Geometry: final body of the model. Coordinates: model frame, mm. Face numbers are marked on the shaded views. A direction names the side the tool comes from. Give positions to 0.01 mm unless a question says otherwise; leave off trailing zeros. Order: outer loops, then holes, each group sorted by start corner. A loop starts at its lowest first (then second) coordinate and runs counter-clockwise, first axis right, second up. Notation, with made-up numbers: (71, -35.5) -> (80, -35.5) arc R16 ccw to (80, -25.5) -> close; hole circle Ø11 at (59, 69). An arc over 180 degrees is marked (long way). One line per question, with ' | ' between items.
Autodesk Inventor part; units mm, degrees
ref_plane "YZ Plane" through (0, 0, 0) normal (1, 0, 0) x (0, 1, 0)
ref_plane "XZ Plane" through (0, 0, 0) normal (0, 1, 0) x (-1, 0, 0)
ref_plane "XY Plane" through (0, 0, 0) normal (0, 0, 1) x (1, 0, 0)
sketch "Sketch1" plane through (0, 0, 0) normal (0, 1, 0) x (-1, 0, 0)
  line L0 (0, 0) -> (75, 0)
  line L1 (75, 0) -> (75, -75)
  line L2 (75, -75) -> (0, -75)
  line L3 (0, -75) -> (0, 0)
  dimension "d0" = 75
  dimension "d1" = 75
extrude "Extrusion1" add sketch "Sketch1" along normal blind 3.5
sketch "Sketch2" plane through (0, 3.5, 0) normal (0, 1, 0) x (1, 0, 0)
  line L0 (-75, 0) -> (0, 0)
  line L1 (0, 0) -> (0, 75)
  line L2 (0, 75) -> (-75, 75)
  line L3 (-75, 75) -> (-75, 0)
  line L4 (-75, 75) -> (-75, 0)
  line L5 (0, 0) -> (0, 75)
  line L6 (-5, 5) -> (-75, 5)
  line L7 (-70, 75) -> (-70, 0)
  circle A0 centre (-70, 37.5) radius 2.5
  circle A1 centre (-5, 37.5) radius 2.5
  line L8 (-75, 37.5) -> (-7.5, 37.5)
  line L9 (-2.5, 37.5) -> (0, 37.5)
  line L10 (-5, 75) -> (-5, 40)
  line L11 (-5, 35) -> (-5, 5)
  dimension "d5" = 5
  dimension "d6" = 5
  dimension "d7" = 5
extrude "Extrusion2" cut sketch "Sketch2" against normal blind 3.5 contours A0 L8 L7 | L7 L8 A0 | A0 L7 L8 | A1 | L7 A0 L8
sketch "Sketch3" plane through (0, 3.5, 0) normal (0, 1, 0) x (1, 0, 0)
  circle A0 centre (-70, 37.5) radius 2.5
  circle A1 centre (-5, 37.5) radius 2.5
  line L0 (-75, 0) -> (0, 0)
  line L1 (0, 0) -> (0, 75)
  line L2 (0, 75) -> (-75, 75)
  line L3 (-75, 75) -> (-75, 0)
  line L4 (-10, 10) -> (-10, 65)
  line L5 (-65, 65) -> (-65, 10)
  line L6 (-65, 65) -> (-65, 75)
  line L7 (0, 75) -> (-75, 75)
  line L8 (-65, 10) -> (-65, 0)
  line L9 (-75, 0) -> (0, 0)
  line L10 (-10, 10) -> (-10, 0)
  line L11 (-10, 65) -> (-10, 75)
  dimension "d10" = 10
extrude "Extrusion3" add sketch "Sketch3" along normal blind 32 contours L8 L5 L6 L2 L11 L4 L10 L0
properties part number "power_suply"
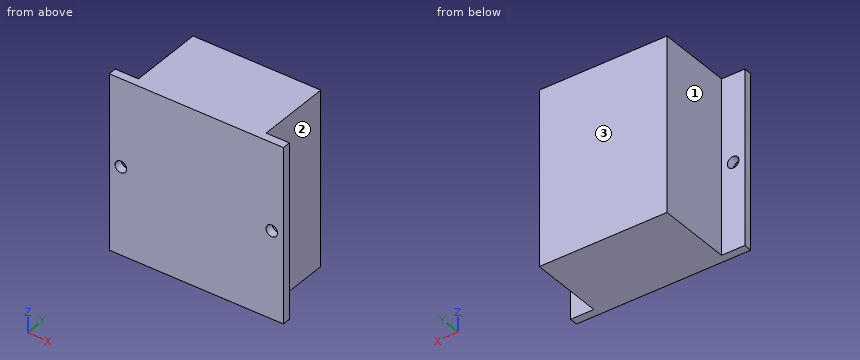
1) Material intervals for probe 1 along X at (y, z) = (0.95, -37.5); probe 2 along Z at (x, y) = (-5, 2); probe 3 along X at (y, z) = (2, -37), sorted ascending. Write a range as from..to.
Check result:
probe 1: x = -75..-72.5, -67.5..-7.5, -2.5..0 | probe 2: z = -75..-40, -35..0 | probe 3: x = -75..-72.45, -67.55..-7.45, -2.55..0
2) Set-up query: the marked faces 1, 2 and 3. Return all of +Z, -Z, +X, -X, +Y, -Y with unobstructed straight access to the full face (end or side cutting, diameter ignored); none if empty.
Check result:
face 1: +Z, -Z, -X, +Y | face 2: +Z, -Z, +X, +Y | face 3: +Z, -Z, +X, -X, +Y
3) Section B-B on x = -70. Return loops of the section in (y, z).
Check result:
outline: (0, -75) -> (3.5, -75) -> (3.5, -40) -> (0, -40) -> close; (0, -35) -> (3.5, -35) -> (3.5, 0) -> (0, 0) -> close
4) Section C-C on y = 28.5. Return loops of the section in (x, z).
Check result:
outline: (-65, -75) -> (-10, -75) -> (-10, 0) -> (-65, 0) -> close
5) Section A-A on z = -37.5. Return loops of the section in (x, y), plus the area to 3 significant figures.
Check result:
outline: (-75, 0) -> (-72.5, 0) -> (-72.5, 3.5) -> (-75, 3.5) -> close; (-67.5, 0) -> (-7.5, 0) -> (-7.5, 3.5) -> (-10, 3.5) -> (-10, 35.5) -> (-65, 35.5) -> (-65, 3.5) -> (-67.5, 3.5) -> close; (-2.5, 0) -> (0, 0) -> (0, 3.5) -> (-2.5, 3.5) -> close | area: 1,990 mm^2
6) Contact query for flat-ended pins moving along their axis: pin 1 Ø5 at (x, z) = (-3.5, -29.5) entering from +Y; pin 2 Ø6 at (x, y) = (-21.5, 4) entering from +Z; pin 3 Ø9.5 at (y, z) = (16.5, -25.5) entering from -X; pin 4 Ø16 at (y, z) = (17, -19.5) entering from +X. Output: stop coordinate, or through.
Check result:
pin 1: stops at y = 3.5 | pin 2: stops at z = 0 | pin 3: stops at x = -65 | pin 4: stops at x = -10
